Check sheet for the drawn part. Datum: minimum x, y, z corner. Units: mm. Round coordinates to 2 decimals unless told otherwise and drop trailing zeros. Order: outer loops, then holes, each group sorted by start corner. A loop starts at its lowest first (then second) coordinate and runs counter-clockwise, first axis right, second up. Notation, with made-up numbers: (29, -0.5) - (54, -0.5) arc R11 cw to (54, 18.5) - close; hole circle Ø10 at (8, 88). An arc over 180 degrees is marked (long way). Write each question's results on one line, items separated by ' | '.
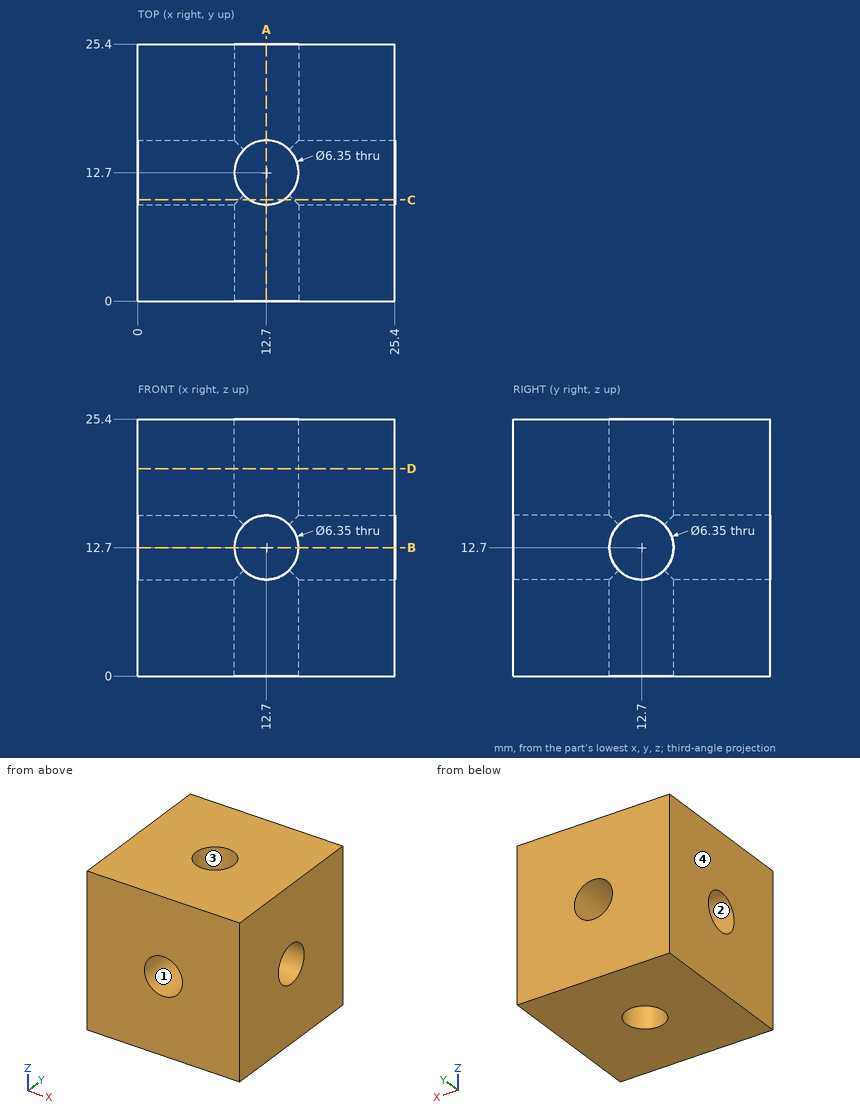
(1) Section check A-A (x = 12.7). Record the cut outline in (y, z) (3 decimals), then the cut area to 3 significant figures.
Answers follow:
outline: (0, 0) - (9.525, 0) - (9.525, 9.525) - (0, 9.525) - close; (0, 15.875) - (9.525, 15.875) - (9.525, 25.4) - (0, 25.4) - close; (15.875, 0) - (25.4, 0) - (25.4, 9.525) - (15.875, 9.525) - close; (15.875, 15.875) - (25.4, 15.875) - (25.4, 25.4) - (15.875, 25.4) - close | area: 363 mm²
(2) Section check D-D (z = 20.5). Record the cut outline in (x, y) (3 decimals).
Answers follow:
outline: (0, 0) - (25.4, 0) - (25.4, 25.4) - (0, 25.4) - close; hole circle Ø6.35 at (12.7, 12.7)
(3) Draft check along X on the marked faces 1, 2, 3 and 4. Enter one of: released by +X, released by -X, zero draft, split by the parting line, or undercut.
Answers follow:
face 1: undercut | face 2: zero draft | face 3: undercut | face 4: released by -X
(4) Section check C-C (y = 10). Record the cut outline in (x, z) (3 decimals), then the cut area to 3 significant figures.
Answers follow:
outline: (0, 0) - (11.029, 0) - (11.029, 10) arc R3.175 cw to (10, 11.029) - (0, 11.029) - close; (0, 14.371) - (10, 14.371) arc R3.175 cw to (11.029, 15.4) - (11.029, 25.4) - (0, 25.4) - close; (14.371, 0) - (25.4, 0) - (25.4, 11.029) - (15.4, 11.029) arc R3.175 cw to (14.371, 10) - close; (14.371, 15.4) arc R3.175 cw to (15.4, 14.371) - (25.4, 14.371) - (25.4, 25.4) - (14.371, 25.4) - close | area: 484 mm²
(5) Material ranges on line 1 (Y direction, x = 12.7, z = 22.75) (3 decimals), recorded low to high.
Answers follow:
line 1: 0 to 9.525, 15.875 to 25.4
